Answer from the drawing. Dimensions are ordinates in mm from the lowest x, y and z of the part. A direction names the side the tool comes from. Give positions to 0.01 mm unless a question says otherwise; leave off trailing zeros. Order: outer loops, then holes, each group sorted by start corner. A loop starts at its lowest first (then second) coordinate and runs counter-clockwise, first axis right, second up. Notation, with made-up numbers: (73.25, -26) - (99.25, -26) arc R15 ccw to (99.25, -6) - close; hole circle Ø10 at (-6.75, -6). An arc over 180 degrees is marked (long way). Answer in a Markdown table with one row per item. Add a question column.
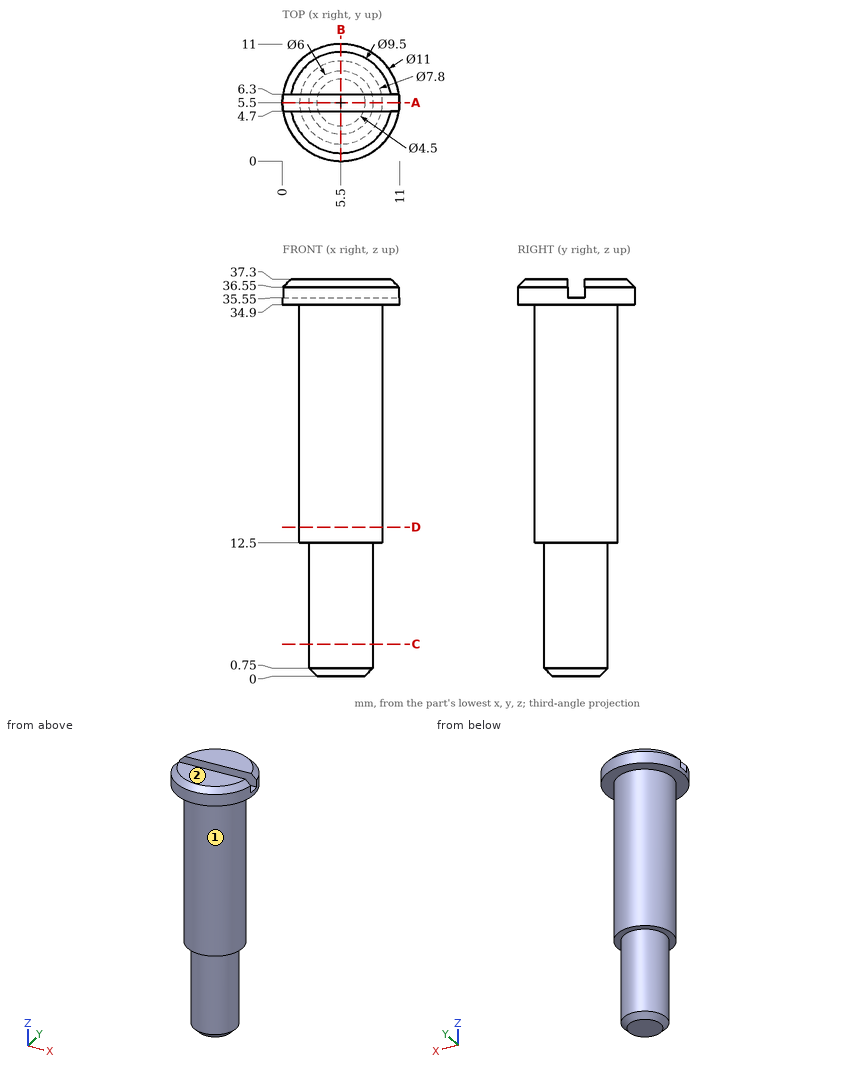
(1) Find section D-D, the plane z = 14. Write down the section's boundary in (x, y), plus the area to 3 significant figures.
(2) Each of these flat-tipped pins is pushed along its axis until it touches: P1, Ø3, axis at x = 1.5, y = 6, coming from the -Z side; P2, Ø1.4, axis at x = 4.5, z = 36, coming from the -Y side; P3, Ø1, axis at x = 2.5, y = 4, coming from the -Z side. Where does it stop, or does it pass through?
(3) Find section B-B, the plane x = 5.5. Write down the section's boundary in (y, z).
(4) For the marked faces 1 and 2, determine the directions among +Z, -Z, +X, -X, +Y, -Y from which every point of the face is accessible in a straight line to the end or side of a thin tool.
(5) Find section A-A, the plane y = 5.5. Write down the section's boundary in (x, z).
(6) Find section C-C, the plane z = 3. Write down the section's boundary in (x, y), plus the area to 3 significant figures.
(7) Straight lines are drawn through the part: line 1 (Y direction, x = 3, z = 21.5); line 2 (Y direction, x = 5.5, z = 16); line 3 (Z direction, x = 7.5, y = 5). For each, find the intervals that lie inside material, in ascending order.
Answer key:
| question | item | result |
|---|---|---|
| 1 | outline | circle Ø7.8 at (5.5, 5.5) |
| 1 | area | 47.8 mm² |
| 2 | P1 | z = 0.28 |
| 2 | P2 | y = 0.01 |
| 2 | P3 | z = 0.6 |
| 3 | outline | (0, 34.9) - (1.6, 34.9) - (1.6, 12.5) - (2.5, 12.5) - (2.5, 0.75) - (3.25, 0) - (7.75, 0) - (8.5, 0.75) - (8.5, 12.5) - (9.4, 12.5) - (9.4, 34.9) - (11, 34.9) - (11, 36.55) - (10.25, 37.3) - (6.3, 37.3) - (6.3, 35.55) - (4.7, 35.55) - (4.7, 37.3) - (0.75, 37.3) - (0, 36.55) - close |
| 4 | face 1 | -Z |
| 4 | face 2 | +Z, +X, -X, +Y, -Y |
| 5 | outline | (0, 34.9) - (1.6, 34.9) - (1.6, 12.5) - (2.5, 12.5) - (2.5, 0.75) - (3.25, 0) - (7.75, 0) - (8.5, 0.75) - (8.5, 12.5) - (9.4, 12.5) - (9.4, 34.9) - (11, 34.9) - (11, 35.55) - (0, 35.55) - close |
| 6 | outline | circle Ø6 at (5.5, 5.5) |
| 6 | area | 28.3 mm² |
| 7 | line 1 | 2.51 to 8.49 |
| 7 | line 2 | 1.6 to 9.4 |
| 7 | line 3 | 0 to 35.55 |
